Answer from the drawing. Dimensions are ordinates in mm from the lowest x, y and z of the part. A direction names the side the tool comes from. Round coordinates to 2 decimals unless told otherwise and drop trailing zeros. Loops run counter-clockwise (first coordinate to the right, second up) from the corner with the lowest first, then second, coordinate; pieces in that order, holes last.
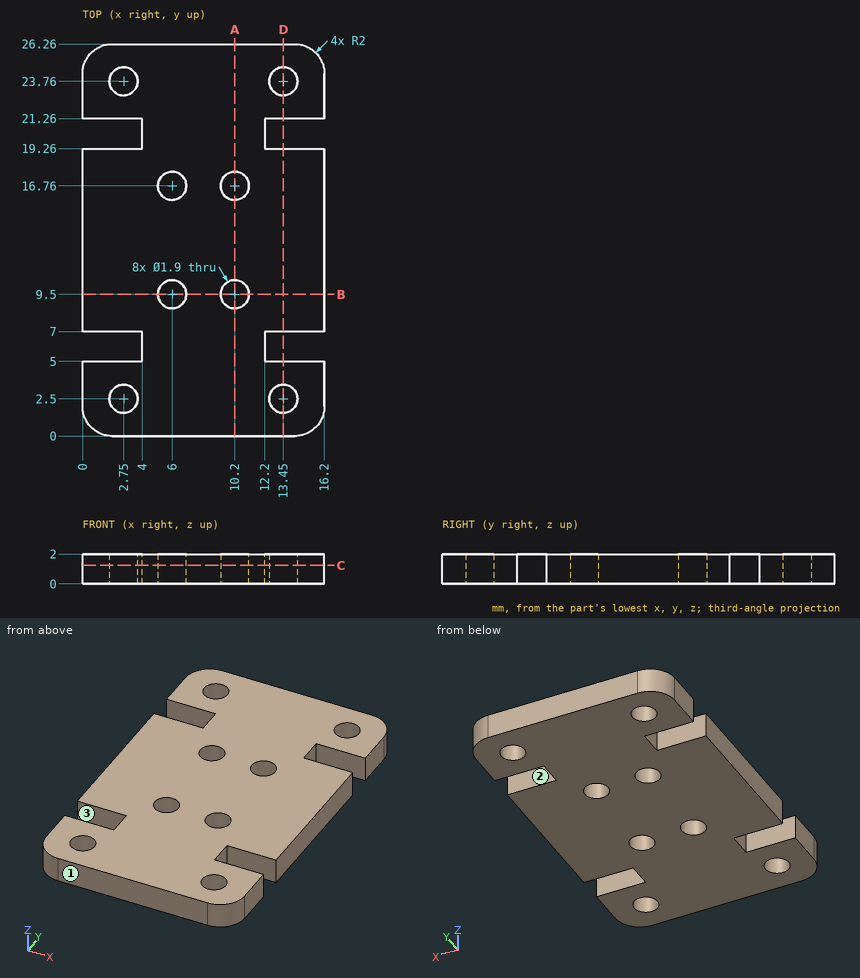
1. Find section B-B (y = 9.5). Write down the section's boundary in (x, z).
Answer key:
outline: (0, 0) - (5.05, 0) - (5.05, 2) - (0, 2) - close; (6.95, 0) - (9.25, 0) - (9.25, 2) - (6.95, 2) - close; (11.15, 0) - (16.2, 0) - (16.2, 2) - (11.15, 2) - close
2. Which of the six approach directions +Z, -Z, +X, -X, +Y, -Y give full straight-line access (tool end or side, diameter ignored) to the marked faces 1, 2 and 3?
Answer key:
face 1: +Z, -Z, +X, -X, -Y
face 2: +Z, -Z, +X
face 3: +Z, -Z, -X
3. Given pin 1 (1 mm diameter, centred on y = 6, z = 1, fed in from +X), flat-ended and moving along its own axis, determine where the tip first touches the part or whether it passes through.
Answer key:
pin 1: stops at x = 12.2
4. Find section A-A (x = 10.2). Write down the section's boundary in (y, z).
Answer key:
outline: (0, 0) - (8.55, 0) - (8.55, 2) - (0, 2) - close; (10.45, 0) - (15.81, 0) - (15.81, 2) - (10.45, 2) - close; (17.71, 0) - (26.26, 0) - (26.26, 2) - (17.71, 2) - close
5. Consider probe 1 along Y at (x, z) = (2.75, 1.15); probe 2 along X at (y, z) = (2.5, 1.15); probe 3 along Y at (x, z) = (6, 0.55). Determine where each line is inside the solid, lowest interval first.
Answer key:
probe 1: y = 0 to 1.55, 3.45 to 5, 7 to 19.26, 21.26 to 22.81, 24.71 to 26.26
probe 2: x = 0 to 1.8, 3.7 to 12.5, 14.4 to 16.2
probe 3: y = 0 to 8.55, 10.45 to 15.81, 17.71 to 26.26
6. Find section C-C (z = 1.25). Give the number of separate pieces and of enclosed holes in the cut face, then the cut area to 3 significant figures.
Answer key:
separate pieces: 1
enclosed holes: 8
area: 367 mm2
7. Find section D-D (x = 13.45). Write down the section's boundary in (y, z), then the cut area to 3 significant figures.
Answer key:
outline: (0, 0) - (1.55, 0) - (1.55, 2) - (0, 2) - close; (3.45, 0) - (5, 0) - (5, 2) - (3.45, 2) - close; (7, 0) - (19.26, 0) - (19.26, 2) - (7, 2) - close; (21.26, 0) - (22.81, 0) - (22.81, 2) - (21.26, 2) - close; (24.71, 0) - (26.26, 0) - (26.26, 2) - (24.71, 2) - close
area: 36.9 mm2
